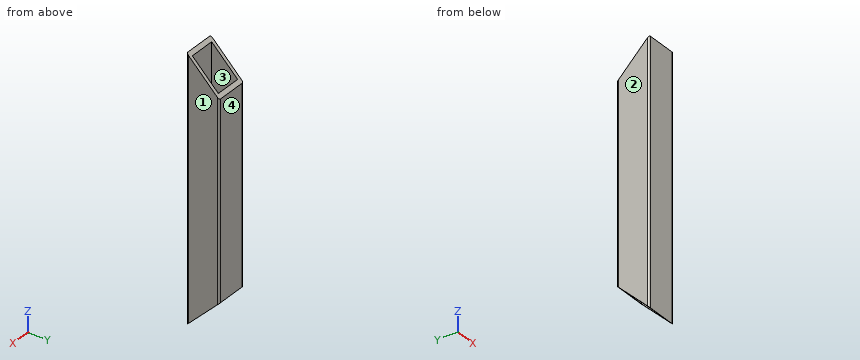
```python
from build123d import *

# Parameters (mm, degrees)
SKETCH_11_W          = 8
SKETCH_11_H          = 8
MEMBER_10_10_1_DEPTH = 80
CUT_EXTRUDE_1_DEPTH  = 5


with BuildPart() as part:
    # 草图11 → Member 10_10_1 (new body)
    with BuildSketch(Plane.YX):
        with BuildLine():
            Line((-4.5, -5), (4.5, -5))
            ThreePointArc((4.5, -5), (4.853553391, -4.853553391), (5, -4.5))
            Line((5, -4.5), (5, 4.5))
            ThreePointArc((5, 4.5), (4.853553391, 4.853553391), (4.5, 5))
            Line((4.5, 5), (-4.5, 5))
            ThreePointArc((-4.5, 5), (-4.853553391, 4.853553391), (-5, 4.5))
            Line((-5, 4.5), (-5, -4.5))
            ThreePointArc((-5, -4.5), (-4.853553391, -4.853553391), (-4.5, -5))
        make_face()
        Rectangle(SKETCH_11_W, SKETCH_11_H, mode=Mode.SUBTRACT)
    extrude(amount=MEMBER_10_10_1_DEPTH)

    # 草图12 → 切除-拉伸1 (cut, symmetric)
    with BuildSketch(Plane(origin=(0, 0, 0), x_dir=(0, 0, -1), z_dir=(1, 0, 0))):
        Polygon((0, -5), (0, 5), (10, 5), align=None)
        Polygon((80, -5), (80, 5), (70, 5), align=None)
    extrude(amount=CUT_EXTRUDE_1_DEPTH, both=True, mode=Mode.SUBTRACT)


solid = part.part
```
The listing builds one solid part. Answer for the finished solid, in the listing's coordinates (mm). Face numbers are marked on the shaded views. Give positions to 0.01 mm unless a question says otherwise; leave off trailing zeros. Loops run counter-clockwise (first coordinate to the right, second up) from the corner with the lowest first, then second, coordinate; pieces in that order, holes last. Notation, with made-up numbers: (74, 44.25) - (91, 44.25) arc R26 cw to (91, 77.25) - close; hole circle Ø6 at (41, 29). An arc over 180 degrees is marked (long way). Return JSON: item names as keys, results as strings. Group by question number.
1. Find section A-A (y = -1.5). Write down the section's boundary in (x, z), then the cut area to 3 significant figures.
2. Find section C-C (z = -47). Write down the section's boundary in (x, y).
3. Find section B-B (x = 1.25). Write down the section's boundary in (y, z), then the cut area to 3 significant figures.
4. Determine the mould class of the marked faces 1, 2, 3 and 4 for opening direction X: pulls with the +X half, pulls with the -X half, needs draft (parallel to the pull), parting line crosses it, or undercut.
5. Given pin 1 Ø5 at (x, y) = (3.5, 3) entering from -Z; pin 2 Ø6 at (x, y) = (-4, 0) entering from -Z, each flat-ended and moving along its own axis, determine where each tip first touches the part or whether it passes through.
6. Straight lines are drawn through the part: line 1 (Y direction, x = 0.75, z = -42.5); line 2 (Y direction, x = -3.25, z = -73). For each, find the intervals that lie inside material, in ascending order. Write a range as [from, to].
Verdict:
{
 "1": {"outline": "(-5, -76.5) - (-4, -76.5) - (-4, -3.5) - (-5, -3.5) - close; (4, -76.5) - (5, -76.5) - (5, -3.5) - (4, -3.5) - close", "area": "146 mm^2"},
 "2": {"outline": "(-5, -4.5) arc R0.5 ccw to (-4.5, -5) - (4.5, -5) arc R0.5 ccw to (5, -4.5) - (5, 4.5) arc R0.5 ccw to (4.5, 5) - (-4.5, 5) arc R0.5 ccw to (-5, 4.5) - close; hole (-4, -4) - (4, -4) - (4, 4) - (-4, 4) - close"},
 "3": {"outline": "(-5, -80) - (-4, -79) - (-4, -1) - (-5, 0) - close; (4, -71) - (5, -70) - (5, -10) - (4, -9) - close", "area": "140 mm^2"},
 "4": {"face 1": "pulls with the +X half", "face 2": "pulls with the -X half", "face 3": "undercut", "face 4": "needs draft"},
 "5": {"pin 1": "stops at z = -74.45", "pin 2": "stops at z = -78"},
 "6": {"line 1": "y = [-5, -4], [4, 5]", "line 2": "y = [-5, -4]"}
}
